Print and shaded views of the part. All mm, measured from the part's lowest x, y and z. A direction names the side the tool comes from. Round coordinates to 2 decimals unless told otherwise and drop trailing zeros. Loops run counter-clockwise (first coordinate to the right, second up) from the corner with the lowest first, then second, coordinate; pieces in that order, holes last. Notation, with made-up numbers: (42, -25.75) - (97, -25.75) arc R21 cw to (97, 4.25) - close; hole circle Ø2 at (-40, 64.25). An arc over 180 degrees is marked (long way). Use one line per item in the form item = value.
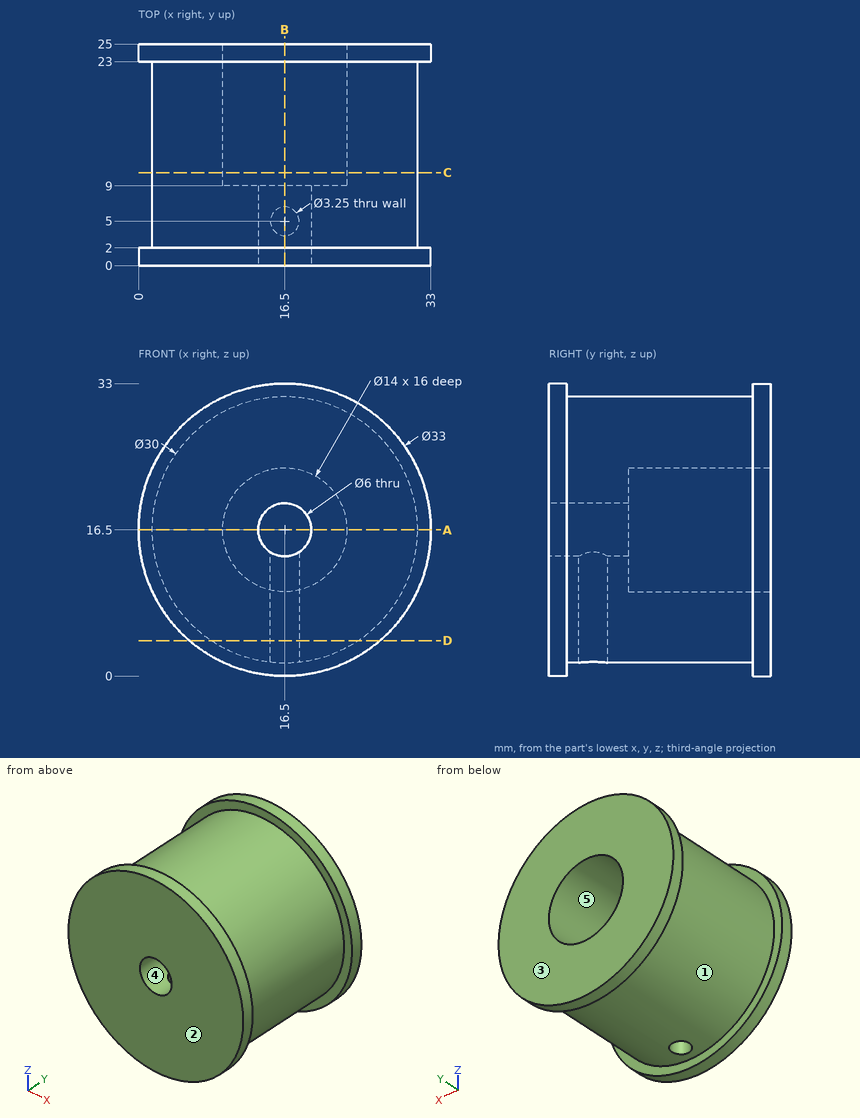
1) Slice it at D-D (z = 4). Write the cut outline in (x, y) (3 decimals).
Report:
outline = (5.73, 0) - (27.27, 0) - (27.27, 2) - (24.792, 2) - (24.792, 23) - (27.27, 23) - (27.27, 25) - (5.73, 25) - (5.73, 23) - (8.208, 23) - (8.208, 2) - (5.73, 2) - close; hole circle Ø3.25 at (16.5, 5)
2) Tool access for the marked faces 4 and 5: list every direction of +Z, -Z, +X, -X, +Y, -Y with a clear straight run to the whole face (end or side of a thin tool).
Report:
face_4 = +Y, -Y
face_5 = +Y
3) Slice it at A-A (z = 16.5). Write the cut outline in (x, y), plus the area to 3 significant figures.
Report:
outline = (0, 0) - (13.5, 0) - (13.5, 9) - (9.5, 9) - (9.5, 25) - (0, 25) - (0, 23) - (1.5, 23) - (1.5, 2) - (0, 2) - close; (19.5, 0) - (33, 0) - (33, 2) - (31.5, 2) - (31.5, 23) - (33, 23) - (33, 25) - (23.5, 25) - (23.5, 9) - (19.5, 9) - close
area = 484 mm^2
4) Two-plate mould, pull along Y, no slides. Class the marked faces 1, 2 and 3: +Y half, -Y half, draft (parallel to the pull), parting line (faces both ways), or undercut.
Report:
face_1 = undercut
face_2 = -Y half
face_3 = +Y half
5) Slice it at C-C (y = 10.5). Write the cut outline in (x, z), plus the area to 3 significant figures.
Report:
outline = circle Ø30 at (16.5, 16.5); hole circle Ø14 at (16.5, 16.5)
area = 553 mm^2
6) Flat gauge pins, fed straight in: pin 1 (5 mm diameter, centred on x = 16.5, y = 5, fed in from -Z); pin 2 (1 mm diameter, centred on y = 22, z = 29, fed in from +X); pin 3 (5 mm diameter, centred on y = 17, z = 12, fed in from +X); pin 4 (16.5 mm diameter, centred on x = 16.5, z = 16.5, fed in from +Y). Where does each tip first touch, or does it go through?
Report:
pin_1 = 1.5
pin_2 = 25.5
pin_3 = 31.37
pin_4 = 25
7) Drill centre lines: probe 1 along Y at (x, z) = (16.5, 6.75) (3 decimals); probe 2 along Z at (x, y) = (16.5, 13.5); probe 3 along Z at (x, y) = (16.5, 4). Where is each one in solid material? Low to high.
Report:
probe_1 = 0 to 3.375, 6.625 to 25
probe_2 = 1.5 to 9.5, 23.5 to 31.5
probe_3 = 19.5 to 31.5
8) Slice it at B-B (x = 16.5). Write the cut outline in (y, z) (3 decimals).
Report:
outline = (0, 0) - (2, 0) - (2, 1.5) - (3.375, 1.5) - (3.375, 13.5) - (0, 13.5) - close; (0, 19.5) - (9, 19.5) - (9, 23.5) - (25, 23.5) - (25, 33) - (23, 33) - (23, 31.5) - (2, 31.5) - (2, 33) - (0, 33) - close; (6.625, 1.5) - (23, 1.5) - (23, 0) - (25, 0) - (25, 9.5) - (9, 9.5) - (9, 13.5) - (6.625, 13.5) - close
